Source: CAD feature listing. Evaluate the final solid. Frame: model axes, mm. A direction names the side the tool comes from. Round coordinates to 2 decimals unless told otherwise and drop trailing zeros. Order: outer loops, then holes, each group sorted by start corner. A loop starts at its lowest first (then second) coordinate and runs counter-clockwise, first axis right, second up. Notation, with made-up numbers: (62, 51) -> (73, 51) arc R26 ccw to (73, 78) -> close; hole circle Ø4 at (38.5, 85). An arc over 180 degrees is marked (long way). One line per item, written item: value. Start each with the question number.
1) Ray query, L1, parallel to Z at x = 6.25, y = 87 (3 decimals); L2, parallel to X at y = 118.5, z = -8.5 (3 decimals); L3, parallel to Y at x = 12.7, z = 11.3 (3 decimals). Return the intervals inside material, ascending.
2) Section C-C (y = 112). Return the cut outline in (x, z) (3 decimals), and give its area (3 significant figures).
3) Section B-B (y = 0). Return the cut outline in (x, z) (3 decimals), and give its area (3 significant figures).
4) Reachability of faces 4 (the face through (3.175, 90, 0)), 5 (the face through (15, 2, 12.7)), 6 (the face through (1.61, 10.79, -7.714)) from +Z, -Z, +X, -X, +Y, -Y: full face, straight path, thin tool, end or side. Return the list, or none.
5) Section A-A (x = 19). Return the cut outline in (y, z) (3 decimals), and give its area (3 significant figures).
6) Mould query, pull axis X, two halves, no side actions, for faces 1 (the face through (0, 2, -11)), 2 (the face through (16, -2, -9.525)), 3 (the face through (24, 172.085, 0)). Classes: pulls with the +X half, pulls with the -X half, needs draft (parallel to the pull), parting line crosses it, or undercut.
```python
from build123d import *

# Parameters (mm, degrees)
SKETCH1_W           = 25.4
SKETCH1_H           = 25.4
SKETCH1_W_2         = 19.05
SKETCH1_H_2         = 19.05
BOSS_EXTRUDE1_DEPTH = 172.085
SKETCH2_W           = 19.05
SKETCH2_H           = 25.4
CUT_EXTRUDE1_DEPTH  = 3.175
SKETCH3_R           = 2.4892
SKETCH3_R_2         = 5.55625
CUT_EXTRUDE2_DEPTH  = 26.4
FILLET1_R           = 6.35


with BuildPart() as part:
    # Sketch1 → Boss-Extrude1 (new body, symmetric)
    with BuildSketch(Plane(origin=(0, 0, 0), x_dir=(1, 0, 0), z_dir=(0, 1, 0))):
        with Locations((12.7, 0)):
            Rectangle(SKETCH1_W, SKETCH1_H)
        with Locations((12.7, 0)):
            Rectangle(SKETCH1_W_2, SKETCH1_H_2, mode=Mode.SUBTRACT)
    extrude(amount=BOSS_EXTRUDE1_DEPTH, both=True)

    # Sketch2 → Cut-Extrude1 (cut)
    with BuildSketch(Plane.ZY):
        Rectangle(SKETCH2_W, SKETCH2_H)
    extrude(amount=-CUT_EXTRUDE1_DEPTH, mode=Mode.SUBTRACT)

    # Sketch3 → Cut-Extrude2 (cut, through all)
    with BuildSketch(Plane(origin=(0, 0, -12.7), x_dir=(-1, 0, 0), z_dir=(0, 0, -1))):
        with Locations((-12.7, -159.385)):
            Circle(SKETCH3_R)
        with Locations((-12.7, -133.985)):
            Circle(SKETCH3_R)
        with Locations((-9.525, 0)):
            Circle(SKETCH3_R_2)
    cut_extrude2 = extrude(amount=-CUT_EXTRUDE2_DEPTH, mode=Mode.SUBTRACT)

    # Mirror1: Cut-Extrude2 across plane
    add(cut_extrude2.mirror(Plane.ZX), mode=Mode.SUBTRACT)

    # Fillet1
    fillet1_edges = [part.edges().sort_by_distance(p)[0] for p in [
        (1.5875, 12.7, -9.525),
        (1.5875, -12.7, -9.525),
        (1.5875, -12.7, 9.525),
        (1.5875, 12.7, 9.525),
    ]]
    fillet(fillet1_edges, radius=FILLET1_R)


solid = part.part
```
Findings:
1. L1: -12.7 to -9.525, 9.525 to 12.7
1. L2: 0 to 3.175, 22.225 to 25.4
1. L3: -172.085 to -161.874, -156.896 to -136.474, -131.496 to -4.56, 4.56 to 131.496, 136.474 to 156.896, 161.874 to 172.085
2. outline: (0, -12.7) -> (25.4, -12.7) -> (25.4, 12.7) -> (0, 12.7) -> close; hole (3.175, -9.525) -> (22.225, -9.525) -> (22.225, 9.525) -> (3.175, 9.525) -> close
2. area: 282 mm2
3. outline: (0, -12.7) -> (3.969, -12.7) -> (3.969, -9.525) -> (0, -9.525) -> close; (0, 9.525) -> (3.969, 9.525) -> (3.969, 12.7) -> (0, 12.7) -> close; (15.081, -12.7) -> (25.4, -12.7) -> (25.4, 12.7) -> (15.081, 12.7) -> (15.081, 9.525) -> (22.225, 9.525) -> (22.225, -9.525) -> (15.081, -9.525) -> close
3. area: 151 mm2
4. face 4: +Y, -Y
4. face 5: +Z, +X, -X, +Y, -Y
4. face 6: -X
5. outline: (-172.085, -12.7) -> (172.085, -12.7) -> (172.085, -9.525) -> (-172.085, -9.525) -> close; (-172.085, 9.525) -> (172.085, 9.525) -> (172.085, 12.7) -> (-172.085, 12.7) -> close
5. area: 2,190 mm2
6. face 1: pulls with the -X half
6. face 2: undercut
6. face 3: needs draft
